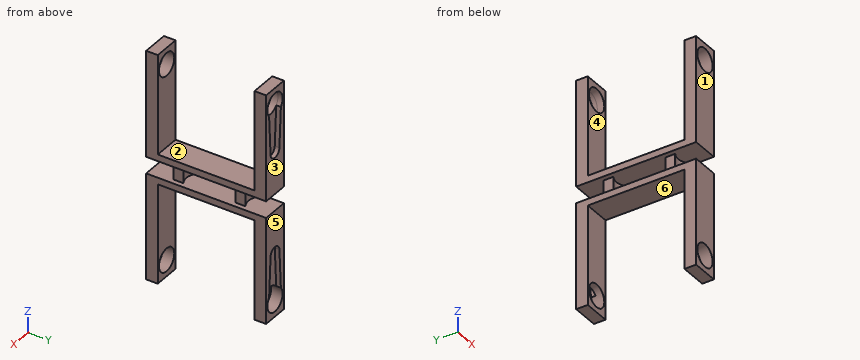
from build123d import *

# Parameters (mm, degrees)
SKETCH2_W            = 8
SKETCH2_H            = 36.15
BOSS_EXTRUDE2_DEPTH  = 2
SKETCH11_W           = 8
SKETCH11_H           = 3.5
BOSS_EXTRUDE8_DEPTH  = 30
CUT_EXTRUDE1_DEPTH   = 1.4
BOSS_EXTRUDE9_DEPTH  = 5
SKETCH15_W           = 8
SKETCH15_H           = 36.15
BOSS_EXTRUDE10_DEPTH = 2
SKETCH16_W           = 8
SKETCH16_H           = 3.5
BOSS_EXTRUDE11_DEPTH = 30
CUT_EXTRUDE4_DEPTH   = 1.4
SKETCH22_R           = 3.45
CUT_EXTRUDE6_DEPTH   = 53.440272523
SKETCH23_R           = 3.45
CUT_EXTRUDE7_DEPTH   = 53.440272523


with BuildPart() as part:
    # Sketch2 → Boss-Extrude2 (new body)
    with BuildSketch(Plane.XY):
        with Locations((-4.61160109, -17.108451256)):
            Rectangle(SKETCH2_W, SKETCH2_H)
    extrude(amount=BOSS_EXTRUDE2_DEPTH)

    # Sketch11 → Boss-Extrude8 (add)
    with BuildSketch(Plane.XY.offset(2)):
        with Locations((-4.61160109, -0.783451256)):
            Rectangle(SKETCH11_W, SKETCH11_H)
        with Locations((-4.61160109, -33.433451256)):
            Rectangle(SKETCH11_W, SKETCH11_H)
    extrude(amount=BOSS_EXTRUDE8_DEPTH)

    # Sketch12 → Cut-Extrude1 (cut)
    with BuildSketch(Plane(origin=(0, 0.966548744, 0), x_dir=(1, 0, 0), z_dir=(0, 1, 0))):
        with BuildLine():
            Line((-2.614580209, -12.840878033), (-1.96160109, -24.790927797))
            ThreePointArc((-1.96160109, -24.790927797), (-4.61160109, -30.45), (-7.26160109, -24.790927797))
            Line((-7.26160109, -24.790927797), (-6.60862197, -12.840878033))
            ThreePointArc((-6.60862197, -12.840878033), (-4.61160109, -10.95), (-2.614580209, -12.840878033))
        make_face()
    extrude(amount=-CUT_EXTRUDE1_DEPTH, mode=Mode.SUBTRACT)

    # Sketch14 → Boss-Extrude9 (add)
    with BuildSketch(Plane(origin=(0, 0, 0), x_dir=(-1, 0, 0), z_dir=(0, 0, -1))):
        with BuildLine():
            Line((2.11160109, -6.31186882), (2.11160109, -9.31186882))
            add(Edge.make_bspline(
                [(2.11160109, -9.31186882), (4.5926591, -7.783279628), (7.11160109, -9.254861144)],
                knots=[0, 0, 0, 1, 1, 1], degree=2))
            Line((7.11160109, -9.254861144), (7.11160109, -6.254861144))
            add(Edge.make_bspline(
                [(2.11160109, -6.31186882), (4.628213222, -7.783477077), (7.11160109, -6.254861144)],
                knots=[0, 0, 0, 1, 1, 1], degree=2))
        make_face()
        with BuildLine():
            Line((2.11160109, -24.982494275), (2.11160109, -27.982494275))
            add(Edge.make_bspline(
                [(2.11160109, -27.982494275), (4.610423864, -26.431016384), (7.11160109, -27.889739685)],
                knots=[0, 0, 0, 1, 1, 1], degree=2))
            Line((7.11160109, -27.889739685), (7.11160109, -24.889739685))
            add(Edge.make_bspline(
                [(2.11160109, -24.982494275), (4.664129849, -26.440271128), (7.11160109, -24.889739685)],
                knots=[0, 0, 0, 1, 1, 1], degree=2))
        make_face()
    extrude(amount=BOSS_EXTRUDE9_DEPTH)

    # Sketch15 → Boss-Extrude10 (add)
    with BuildSketch(Plane(origin=(0, 0, -5), x_dir=(-1, 0, 0), z_dir=(0, 0, -1))):
        with Locations((4.61160109, -17.108451256)):
            Rectangle(SKETCH15_W, SKETCH15_H)
    extrude(amount=BOSS_EXTRUDE10_DEPTH)

    # Sketch16 → Boss-Extrude11 (add)
    with BuildSketch(Plane(origin=(0, 0, -7), x_dir=(-1, 0, 0), z_dir=(0, 0, -1))):
        with Locations((4.61160109, -0.783451256)):
            Rectangle(SKETCH16_W, SKETCH16_H)
        with Locations((4.61160109, -33.433451256)):
            Rectangle(SKETCH16_W, SKETCH16_H)
    extrude(amount=BOSS_EXTRUDE11_DEPTH)

    # Sketch20 → Cut-Extrude4 (cut)
    with BuildSketch(Plane(origin=(0, 0.966548744, 0), x_dir=(1, 0, 0), z_dir=(0, 1, 0))):
        with BuildLine():
            Line((-6.60862197, 17.840878033), (-7.26160109, 29.790927797))
            ThreePointArc((-7.26160109, 29.790927797), (-4.61160109, 35.45), (-1.96160109, 29.790927797))
            Line((-1.96160109, 29.790927797), (-2.614580209, 17.840878033))
            ThreePointArc((-2.614580209, 17.840878033), (-4.61160109, 15.95), (-6.60862197, 17.840878033))
        make_face()
    extrude(amount=-CUT_EXTRUDE4_DEPTH, mode=Mode.SUBTRACT)

    # Sketch22 → Cut-Extrude6 (cut, through all)
    with BuildSketch(Plane(origin=(0, 0.966548744, 0), x_dir=(1, 0, 0), z_dir=(0, 1, 0))):
        with Locations(Location((-4.61160109, -27, 0), (0, 0, 270))):
            Circle(SKETCH22_R)
    extrude(amount=-CUT_EXTRUDE6_DEPTH, mode=Mode.SUBTRACT)

    # Sketch23 → Cut-Extrude7 (cut, through all)
    with BuildSketch(Plane(origin=(0, 0.966548744, 0), x_dir=(1, 0, 0), z_dir=(0, 1, 0))):
        with Locations(Location((-4.61160109, 32, 0), (0, 0, 219.814997755))):
            Circle(SKETCH23_R)
    extrude(amount=-CUT_EXTRUDE7_DEPTH, mode=Mode.SUBTRACT)


solid = part.part
Geometry check sheet. Reference: the model listing, model coordinates, mm. Face numbers are marked on the shaded views. A direction names the side the tool comes from. Round coordinates to 2 decimals unless told otherwise and drop trailing zeros. Loops run counter-clockwise (first coordinate to the right, second up) from the corner with the lowest first, then second, coordinate; pieces in that order, holes last.
Item 1: Mould release check, pull along Y, two halves, no side actions. Record for the marked faces 1, 2 and 3: pulls with the +Y half, pulls with the -Y half, needs draft (parallel to the pull), parting line crosses it, or undercut.
Item 2: Cross-section at A-A on y = -19. Record the boundary of the cut face in (x, z), then the cut area to 3 significant figures.
Item 3: Gauge pin test, flat ends, axial feed: pin 1 (2.5 mm diameter, centred on y = -7.5, z = -1.5, fed in from -X); pin 2 (1.5 mm diameter, centred on x = -7, y = -4.5, fed in from +Z); pin 3 (4 mm diameter, centred on x = -3.5, y = -10, fed in from -Z); pin 4 (1 mm diameter, centred on y = -23.5, z = 4, fed in from -X). Record the tip position at first contact, or that the pin passes through.
Item 4: Cross-section at B-B on z = 9.5. Record the boundary of the cut face in (x, y), then the cut area to 3 significant figures.
Item 5: Thickness scan on line 1 (Y direction, x = -2, z = -24.5); line 2 (Z direction, x = -6.25, y = -13); line 3 (X direction, y = 0, z = 27). Record the ranges inside material, lowest first.
Item 6: Cross-section at C-C on z = -32. Record the boundary of the cut face in (x, y), then the cut area to 3 significant figures.
Item 7: Cross-section at D-D on z = 20. Record the boundary of the cut face in (x, y), then the cut area to 3 significant figures.
Item 8: Access from +Z, -Z, +X, -X, +Y, -Y to the whole of each face (thin tool, end or side, straight path). Record for the marked faces 4, 5 and 6.
Answer sheet:
1. face 1: pulls with the -Y half
1. face 2: undercut
1. face 3: pulls with the +Y half
2. outline: (-8.61, -7) - (-0.61, -7) - (-0.61, -5) - (-8.61, -5) - close; (-8.61, 0) - (-0.61, 0) - (-0.61, 2) - (-8.61, 2) - close
2. area: 32.0 mm2
3. pin 1: stops at x = -7.11
3. pin 2: stops at z = 2
3. pin 3: stops at z = -7
3. pin 4: passes through
4. outline: (-8.61, -35.18) - (-0.61, -35.18) - (-0.61, -31.68) - (-8.61, -31.68) - close; (-8.61, -2.53) - (-0.61, -2.53) - (-0.61, 0.97) - (-8.61, 0.97) - close
4. area: 56.0 mm2
5. line 1: y = -35.18 to -31.68, -2.53 to 0.97
5. line 2: z = -7 to -5, 0 to 2
5. line 3: x = -8.61 to -8.06, -1.16 to -0.61
6. outline: (-8.61, -35.18) - (-8.06, -35.18) - (-8.06, -31.68) - (-8.61, -31.68) - close; (-8.61, -2.53) - (-8.06, -2.53) - (-8.06, 0.97) - (-8.61, 0.97) - close; (-1.16, -35.18) - (-0.61, -35.18) - (-0.61, -31.68) - (-1.16, -31.68) - close; (-1.16, -2.53) - (-0.61, -2.53) - (-0.61, 0.97) - (-1.16, 0.97) - close
6. area: 7.70 mm2
7. outline: (-8.61, -35.18) - (-0.61, -35.18) - (-0.61, -31.68) - (-8.61, -31.68) - close; (-8.61, -2.53) - (-0.61, -2.53) - (-0.61, 0.97) - (-2.22, 0.97) - (-2.22, -0.43) - (-7, -0.43) - (-7, 0.97) - (-8.61, 0.97) - close
7. area: 49.3 mm2
8. face 4: +Z, +X, -X
8. face 5: +Z, -Z, +X, -X, +Y
8. face 6: -Z, +X, -X
